```python
from build123d import *

# Parameters (mm, degrees)
SKETCH1_W                     = 40
SKETCH1_H                     = 51.440769906
SKETCH1_R                     = 6.5
SKETCH1_R_2                   = 1.6
BOSS_EXTRUDE1_DEPTH           = 5
M4X0_7_TAPPED_HOLE1_D         = 3.3
CSK_FOR_M3_SFHCS1_D           = 3.2
CSK_FOR_M3_SFHCS1_CSINK_D     = 6.72
CSK_FOR_M3_SFHCS1_CSINK_ANGLE = 90
FILLET1_R                     = 2
M3X0_5_TAPPED_HOLE1_D         = 2.5
M3X0_5_TAPPED_HOLE1_DEPTH     = 16
M3X0_5_TAPPED_HOLE1_TIP       = 0.751075774
LPATTERN1_COUNT               = 2
LPATTERN1_PITCH               = 15


with BuildPart() as part:
    # Sketch1 → Boss-Extrude1 (new body)
    with BuildSketch(Plane.XY):
        with Locations((0, 25.720384953)):
            Rectangle(SKETCH1_W, SKETCH1_H)
        with Locations((0, 25.5)):
            Circle(SKETCH1_R, mode=Mode.SUBTRACT)
        with Locations((0, 14.5)):
            Circle(SKETCH1_R_2, mode=Mode.SUBTRACT)
        with Locations((-9.526279442, 31)):
            Circle(SKETCH1_R_2, mode=Mode.SUBTRACT)
        with Locations(Location((9.526279442, 31, 0), (0, 0, 180))):
            Circle(SKETCH1_R_2, mode=Mode.SUBTRACT)
        with Locations((-12.5, 47.840769906)):
            Circle(SKETCH1_R_2, mode=Mode.SUBTRACT)
        with Locations(Location((12.5, 47.840769906, 0), (0, 0, 180))):
            Circle(SKETCH1_R_2, mode=Mode.SUBTRACT)
    extrude(amount=BOSS_EXTRUDE1_DEPTH)

    # M4x0.7 Tapped Hole1 (through all)
    with Locations(Plane(origin=(0, 0, 0), x_dir=(-1, 0, 0), z_dir=(0, 0, -1))):
        with Locations((-6.581223291, 17), (6.581223291, 17)):
            Hole(M4X0_7_TAPPED_HOLE1_D / 2)

    # CSK for M3 SFHCS1 (through all)
    with Locations(Plane.XY.offset(5)):
        with Locations((-9.526279442, 31), (9.526279442, 31), (0, 14.5)):
            CounterSinkHole(CSK_FOR_M3_SFHCS1_D / 2, CSK_FOR_M3_SFHCS1_CSINK_D / 2, counter_sink_angle=CSK_FOR_M3_SFHCS1_CSINK_ANGLE)

    # Fillet1
    fillet1_edges = [part.edges().sort_by_distance(p)[0] for p in [
        (20, 51.440769906, 2.5),
        (-20, 51.440769906, 2.5),
    ]]
    fillet(fillet1_edges, radius=FILLET1_R)

    # M3x0.5 Tapped Hole1
    with Locations(Plane.XZ):
        with Locations((-16, 2.5), (16, 2.5)):
            Hole(M3X0_5_TAPPED_HOLE1_D / 2, depth=M3X0_5_TAPPED_HOLE1_DEPTH)
            with Locations((0, 0, -(M3X0_5_TAPPED_HOLE1_DEPTH + M3X0_5_TAPPED_HOLE1_TIP / 2))):  # 118° drill point
                Cone(0, M3X0_5_TAPPED_HOLE1_D / 2, M3X0_5_TAPPED_HOLE1_TIP, mode=Mode.SUBTRACT)

    # Sketch34 → M3 Tapped Hole1 (revolve, cut)
    with BuildSketch(Plane(origin=(7.5, 51.440769906, 2.667636596), x_dir=(0, 0, 1), z_dir=(1, 0, 0))):
        Polygon((0, 0), (0, 6), (1.25, 5.248924226), (1.25, 0), align=None)
    m3_tapped_hole1 = revolve(axis=Axis((7.5, 57.790769906, 2.667636596), (0, -1, 0)), mode=Mode.SUBTRACT)

    # LPattern1: M3 Tapped Hole1 ×2
    with Locations(*[(-i * LPATTERN1_PITCH, 0, 0) for i in range(1, LPATTERN1_COUNT)]):
        add(m3_tapped_hole1, mode=Mode.SUBTRACT)


solid = part.part
```
Input: part model. Units: mm. Frame: model coordinates. A direction names the side the tool comes from. Give positions to 0.01 mm unless a question says otherwise; leave off trailing zeros. Loops run counter-clockwise (first coordinate to the right, second up) from the corner with the lowest first, then second, coordinate; pieces in that order, holes last. Notation, with made-up numbers: M -0.5,30.5 L 16.5,30.5 A10 cw 16.5,47.5 Z; hole C 50,48 d1. An arc over 180 degrees is marked long. Answer as CSV lines item,"result". Start each with the question number.
1. Section D-D on x = 4. Return loops of the section in (y, z).
2. Reachability of faces 4 (the face through (13.68, 46.76, 2.46)), 5 (the face through (-15.84, 8.11, 3.74)), 6 (the face through (-6.28, 48.85, 2.4)) from +Z, -Z, +X, -X, +Y, -Y: full face, straight path, thin tool, end or side. Return the list, or none.
3. Pin query (flat end, axial travel): P1, Ø3, axis at x = 16, z = 2.5, coming from the -Y side; P2, Ø2, axis at x = -7.5, z = 2.67, coming from the +Y side. Return the tip coordinate at first contact, or that it passes through.
4. Section A-A on y = 14.5. Return loops of the section in (x, z).
5. Section C-C on y = 31. Return loops of the section in (x, z).
6. Pull-direction query (X, two-part tool) for faces 1 (the face through (-5.69, 18.39, 2.53)), 2 (the face through (0, 51.441, 2)), 3 (the face through (-19.43, 50.84, 2.54)); classes: released by +X, released by -X, zero draft, split by the parting line, or undercut.
7. Section B-B on y = 25.5. Return loops of the section in (x, z).
8. Line query: L1, parallel to X at y = 9.5, z = 2.5; L2, parallel to Y at x = -12.5, z = 3.5; L3, parallel to Y at x = -5.5, z = 1.35. Output: solid intervals per line, ascending.
Computed values:
1,outline,"M 0,0 L 20.38,0 L 20.38,5 L 0,5 Z; M 30.62,0 L 51.44,0 L 51.44,5 L 30.62,5 Z"
2,face 4,"+Z, -Z"
2,face 5,"-Y"
2,face 6,"+Y"
3,P1,"stops at y = 0"
3,P2,"stops at y = 46.04"
4,outline,"M -20,0 L -1.6,0 L -1.6,3.24 L -3.36,5 L -20,5 Z; M 1.6,0 L 20,0 L 20,5 L 3.36,5 L 1.6,3.24 Z; hole C -16,2.5 d2.5; hole C 16,2.5 d2.5"
5,outline,"M -20,0 L -11.13,0 L -11.13,3.24 L -12.89,5 L -20,5 Z; M -7.93,0 L -3.46,0 L -3.46,5 L -6.17,5 L -7.93,3.24 Z; M 3.46,0 L 7.93,0 L 7.93,3.24 L 6.17,5 L 3.46,5 Z; M 11.13,0 L 20,0 L 20,5 L 12.89,5 L 11.13,3.24 Z"
6,face 1,"undercut"
6,face 2,"zero draft"
6,face 3,"released by -X"
7,outline,"M -20,0 L -6.5,0 L -6.5,5 L -20,5 Z; M 6.5,0 L 20,0 L 20,5 L 6.5,5 Z"
8,L1,"x = -20 to -17.25, -14.75 to 14.75, 17.25 to 20"
8,L2,"y = 0 to 46.24, 49.44 to 51.44"
8,L3,"y = 0 to 15.75, 18.25 to 22.04, 28.96 to 51.44"
